Could you check a few things on this model? Use its own coordinates, in mm. Face numbers are marked on the shaded views. A direction names the side the tool comes from. Round coordinates to 2 decimals unless told otherwise and drop trailing zeros. Loops run counter-clockwise (first coordinate to the right, second up) from the corner with the lowest first, then second, coordinate; pieces in that order, holes last. Notation, with made-up numbers: (0, 66) -> (7, 66) arc R16 ccw to (7, 97) -> close; hole circle Ø9 at (76, 19.25). An arc over 180 degrees is marked (long way). One line per item, written item: value.
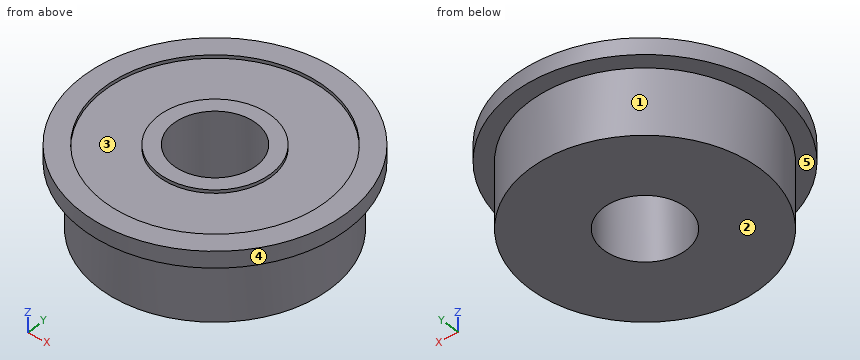
Autodesk Inventor part; units mm, degrees
ref_plane "YZ Plane" through (0, 0, 0) normal (1, 0, 0) x (0, 1, 0)
ref_plane "XZ Plane" through (0, 0, 0) normal (0, 1, 0) x (-1, 0, 0)
ref_plane "XY Plane" through (0, 0, 0) normal (0, 0, 1) x (1, 0, 0)
sketch "Sketch1" plane through (0, 0, 0) normal (0, 0, 1) x (1, 0, 0)
  circle A0 centre (0, 0) radius 5.0674
  circle A1 centre (0, 0) radius 2.5
  circle A2 centre (0, 0) radius 7
  point P0 (0, 0)
  dimension "d0" = 5
  dimension "d1" = 14
extrude "Extrusion1" add sketch "Sketch1" along normal blind 5 contours A0 | A2
sketch "Sketch2" plane through (0, 0, 5) normal (0, 0, 1) x (1, 0, 0)
  circle A0 centre (0, 0) radius 2.5931
  circle A1 centre (0, 0) radius 2.5
  circle A2 centre (0, 0) radius 8
  dimension "d4" = 16
extrude "Extrusion2" add sketch "Sketch2" against normal blind 1 contours A2
sketch "Sketch3" plane through (0, 0, 5) normal (0, 0, 1) x (1, 0, 0)
  circle A0 centre (0, 0) radius 2.5
  circle A1 centre (0, 0) radius 2.5
  circle A2 centre (0, 0) radius 3.4045
  circle A3 centre (0, 0) radius 6.7146
  point P0 (0, 0)
extrude "Extrusion3" cut sketch "Sketch3" against normal blind 0.2 contours A3
properties part number "Flanged Bearing_CPY"
Item 1: If we mould it in two halves opening along X, with no side actions, what happens to the marked faces 3, 4 and 5? For each: released by +X, released by -X, zero draft, split by the parting line, or undercut.
Output:
face 3: undercut
face 4: split by the parting line
face 5: zero draft
Item 2: If we section it at D-D on x = 4.5: List the corners of the cut face in (y, z) for me.
Output:
outline: (-6.61, 4) -> (-5.36, 4) -> (-5.36, 0) -> (5.36, 0) -> (5.36, 4) -> (6.61, 4) -> (6.61, 5) -> (4.98, 5) -> (4.98, 4.8) -> (-4.98, 4.8) -> (-4.98, 5) -> (-6.61, 5) -> close
Item 3: If we section it at A-A on y = 0: List the corners of the cut face in (x, z) for me, plus the area to 3 significant figures.
Output:
outline: (-8, 4) -> (-7, 4) -> (-7, 0) -> (-2.5, 0) -> (-2.5, 5) -> (-3.4, 5) -> (-3.4, 4.8) -> (-6.71, 4.8) -> (-6.71, 5) -> (-8, 5) -> close; (2.5, 0) -> (7, 0) -> (7, 4) -> (8, 4) -> (8, 5) -> (6.71, 5) -> (6.71, 4.8) -> (3.4, 4.8) -> (3.4, 5) -> (2.5, 5) -> close
area: 45.7 mm²
Item 4: I need wall thicknesses on line 1 (Y direction, x = 0, z = 4.9); line 2 (Y direction, x = 0, z = 1.2); line 3 (Z direction, x = -4, y = 6.75). Which ranges of each line are inside material? Lowest first, please. Write a range as from..to.
Output:
line 1: y = -8..-6.71, -3.4..-2.5, 2.5..3.4, 6.71..8
line 2: y = -7..-2.5, 2.5..7
line 3: z = 4..5
Item 5: For the marked faces 1 and 2, which set-ups out of +Z, -Z, +X, -X, +Y, -Y let a thin tool reach every point of the face, with its end or its side?
Output:
face 1: -Z
face 2: -Z, +X, -X, +Y, -Y
Item 6: If we section it at C-C on z = 0.4: List the corners of the cut face in (x, y) for me, plus the area to 3 significant figures.
Output:
outline: circle Ø14 at (0, 0); hole circle Ø5 at (0, 0)
area: 134 mm²
Item 7: Will these pins go through, and if not, where does the flat tip stop? pin 1 Ø1 at (x, z) = (-3, 4) entering from -Y; pin 2 Ø1.5 at (x, z) = (-5, 4.5) entering from -Y.
Output:
pin 1: stops at y = -7.6
pin 2: stops at y = -6.78
